Geometry check sheet. Reference: the model listing, model coordinates, mm. Face numbers are marked on the shaded views. A direction names the side the tool comes from. Round coordinates to 2 decimals unless told otherwise and drop trailing zeros. Loops run counter-clockwise (first coordinate to the right, second up) from the corner with the lowest first, then second, coordinate; pieces in that order, holes last. Notation, with made-up numbers: (19, 44) - (68, 44) arc R18 cw to (68, 65) - close; hole circle Ø5 at (-15.5, -35). An arc over 180 degrees is marked (long way). Answer as CSV lines item,"result". Start each with the question number.
1) Cross-section at A-A on z = 3. Record the boundary of the cut face in (x, y), and give its area (3 significant figures).
2) Cross-section at C-C on y = -20.5. Record the boundary of the cut face in (x, z).
3) Depth check by flat-ended pin: P1, Ø3, axis at y = -6.5, z = -16.5, coming from the +X side; P2, Ø6, axis at x = -30.5, y = -3.5, coming from the -Z side; P3, Ø12, axis at x = 0, z = 0, coming from the +Y side; P4, Ø10, axis at x = 15.5, y = -7.5, coming from the +Z side. Enter the tip coordinate at first touch or a pass-through.
4) Draft check along X on the marked faces 4, 5 and 6. Enter one of: released by +X, released by -X, zero draft, split by the parting line, or undercut.
5) Cross-section at B-B on x = 0. Record the boundary of the cut face in (y, z).
6) Cross-section at D-D on x = -58.5. Record the boundary of the cut face in (y, z), and give its area (3 significant figures).
7) Thickness scan on line 1 along Z through (x, y) = (0, -8.5); line 2 along Z through (x, y) = (-9, -9.5); line 3 along Z through (x, y) = (-26.5, -14). Record the ranges inside material, lowest first.
8) Access from +Z, -Z, +X, -X, +Y, -Y to the whole of each face (thin tool, end or side, straight path). Record for the marked faces 1, 2 and 3.
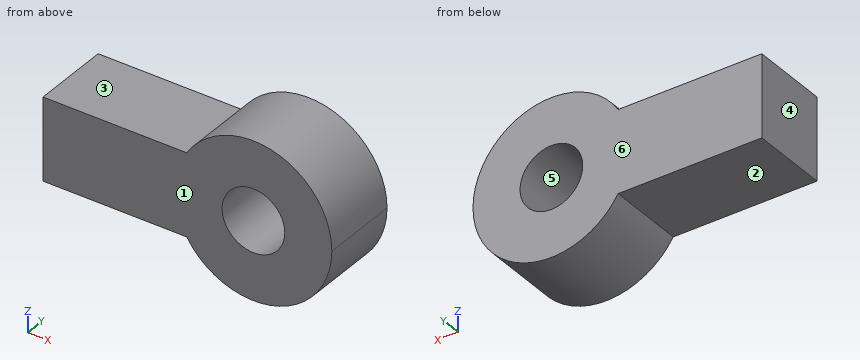
from build123d import *

# Parameters (mm, degrees)
F0_R     = 10
F1_DEPTH = 25


with BuildPart() as f1:
    # F0 (on Front) → F1 (new body)
    with BuildSketch(Plane.XZ):
        with BuildLine():
            Line((-17.164139, 13.151755), (-21.261029, 13.151755))
            ThreePointArc((-21.261029, 13.151755), (-25, 0), (-21.261029, -13.151755))
            Line((-21.261029, -13.151755), (-17.164139, -13.151755))
            Line((-17.164139, -13.151755), (-17.164139, 13.151755))
        make_face()
        with BuildLine():
            ThreePointArc((-21.261029, -13.151755), (-25, 0), (-21.261029, 13.151755))
            Line((-21.261029, 13.151755), (-67.096213, 13.151755))
            Line((-67.096213, 13.151755), (-67.096213, -13.151755))
            Line((-67.096213, -13.151755), (-21.261029, -13.151755))
        make_face()
        with BuildLine():
            ThreePointArc((-21.261029, -13.151755), (6.836457, -24.047097), (25, 0))
            ThreePointArc((25, 0), (6.836457, 24.047097), (-21.261029, 13.151755))
            Line((-21.261029, 13.151755), (-17.164139, 13.151755))
            Line((-17.164139, 13.151755), (-17.164139, -13.151755))
            Line((-17.164139, -13.151755), (-21.261029, -13.151755))
        make_face()
        Circle(F0_R, mode=Mode.SUBTRACT)
    extrude(amount=F1_DEPTH)


solid = f1.part
Answer block:
1,outline,"(-67.1, -25) - (-9.54, -25) - (-9.54, 0) - (-67.1, 0) - close; (9.54, -25) - (24.82, -25) - (24.82, 0) - (9.54, 0) - close"
1,area,"1,820 mm^2"
2,outline,"(-67.1, -13.15) - (-21.26, -13.15) arc R25 ccw (long way) to (-21.26, 13.15) - (-67.1, 13.15) - close; hole circle Ø20 at (0, 0)"
3,P1,"stops at x = 20"
3,P2,"stops at z = -13.15"
3,P3,"passes through"
3,P4,"stops at z = 22.69"
4,face 4,"released by -X"
4,face 5,"undercut"
4,face 6,"zero draft"
5,outline,"(-25, -25) - (0, -25) - (0, -10) - (-25, -10) - close; (-25, 10) - (0, 10) - (0, 25) - (-25, 25) - close"
6,outline,"(-25, -13.15) - (0, -13.15) - (0, 13.15) - (-25, 13.15) - close"
6,area,"658 mm^2"
7,line 1,"z = -25 to -10, 10 to 25"
7,line 2,"z = -23.32 to -4.36, 4.36 to 23.32"
7,line 3,"z = -13.15 to 13.15"
8,face 1,"+Z, -Z, +X, -X, -Y"
8,face 2,"-Z, -X, +Y, -Y"
8,face 3,"+Z, -X, +Y, -Y"
